```python
from build123d import *

# Parameters (mm, degrees)
F0_R         = 38.1
F0_R_2       = 22.86
F1_DEPTH     = 127
F4_DEPTH     = 80.011
F5_T4_DEPTH  = 27.2677982704
F5_S5_R      = 38.1
F5_T6_DEPTH  = 15
F5_S7_R      = 22.86
F5_T8_DEPTH  = 15
F5_T12_DEPTH = 27.2677982704
F5_S13_R     = 38.1
F5_T14_DEPTH = 15
F5_S15_R     = 22.86
F5_T16_DEPTH = 15
F5_T17_DEPTH = 27.2653813946
F5_T19_DEPTH = 27.2653813946


# Not quite as in the source:
# - a fillet or chamfer that OpenCascade refuses, or shapes differently, is made with other operations: its cross-section is extruded or revolved along the edge and cut away or added


with BuildPart() as f1:
    # F0 (on Top) → F1 (new body)
    with BuildSketch(Plane.XY):
        Circle(F0_R)
        Circle(F0_R_2, mode=Mode.SUBTRACT)
    extrude(amount=F1_DEPTH)

    # F3 (on offset) → F4 (cut, through all)
    with BuildSketch(Plane.XZ.offset(41.91)):
        with BuildLine():
            Line((1.3741332924, 44.0691516455), (0, 44.0691516455))
            Line((0, 44.0691516455), (0, 27.1781024958))
            Line((0, 27.1781024958), (0, -6.6039958037))
            Line((0, -6.6039958037), (38.1, -6.6039958037))
            Line((38.1, -6.6039958037), (38.1, 27.1781024958))
            Line((38.1, 27.1781024958), (18.242812226, 27.1781024958))
            ThreePointArc((18.242812226, 27.1781024958), (15.5282171859, 27.7875908663), (13.3347289514, 29.4990556395))
            Line((13.3347289514, 29.4990556395), (1.3741332924, 44.0691516455))
        make_face()
        with BuildLine():
            Line((0, 44.0691516455), (-1.3741332924, 44.0691516455))
            Line((-1.3741332924, 44.0691516455), (-13.3347289514, 29.4990556395))
            ThreePointArc((-13.3347289514, 29.4990556395), (-15.5282171859, 27.7875908663), (-18.242812226, 27.1781024958))
            Line((-18.242812226, 27.1781024958), (-38.1, 27.1781024958))
            Line((-38.1, 27.1781024958), (-38.1, -6.6039958037))
            Line((-38.1, -6.6039958037), (0, -6.6039958037))
            Line((0, -6.6039958037), (0, 27.1781024958))
            Line((0, 27.1781024958), (0, 44.0691516455))
        make_face()
        with BuildLine():
            Line((38.1, 60.9602007953), (38.1, 77.9781024958))
            Line((38.1, 77.9781024958), (1.27, 77.9781024958))
            Line((1.27, 77.9781024958), (1.2895432809, 77.9542953638))
            Line((1.2895432809, 77.9542953638), (13.3347289514, 63.281153939))
            ThreePointArc((13.3347289514, 63.281153939), (15.5282171859, 61.5696891658), (18.242812226, 60.9602007953))
            Line((18.242812226, 60.9602007953), (38.1, 60.9602007953))
        make_face()
        with BuildLine():
            Line((-38.1, 77.9781024958), (-38.1, 60.9602007953))
            Line((-38.1, 60.9602007953), (-18.242812226, 60.9602007953))
            ThreePointArc((-18.242812226, 60.9602007953), (-15.5282171859, 61.5696891658), (-13.3347289514, 63.281153939))
            Line((-13.3347289514, 63.281153939), (-1.2895432809, 77.9542953638))
            Line((-1.2895432809, 77.9542953638), (-1.27, 77.9781024958))
            Line((-1.27, 77.9781024958), (-38.1, 77.9781024958))
        make_face()
        Polygon((-38.1, 131.2988996506), (-38.1, 77.9781024958), (-1.27, 77.9781024958), (-1.2391987117, 77.9781024958), (-0.1262114529, 77.9781024958), (0, 77.9781024958), (1.2391987117, 77.9781024958), (1.27, 77.9781024958), (38.1, 77.9781024958), (38.1, 80.6030047561), (38.1, 131.2988996506), align=None)
    extrude(amount=-F4_DEPTH, mode=Mode.SUBTRACT)

    # F5: fillet of radius 5.08 on 6 edges, made by hand


with BuildPart() as f5_tool2:
    # F5_s3 → F5_t4 (new body)
    with BuildSketch(Plane.XZ.offset(44.0808363055)):
        with BuildLine():
            ThreePointArc((-1.0281164884, 44.0691516455), (1.1435595437, 43.5815609491), (2.8983501313, 42.2123891305))
            Line((2.8983501313, 42.2123891305), (1.3741332924, 44.0691516455))
            Line((1.3741332924, 44.0691516455), (-1.0281164884, 44.0691516455))
        make_face()
    extrude(amount=-F5_T4_DEPTH)

    # F5_s5 → F5_t6 (intersect, symmetric)
    with BuildSketch(Plane.XY.offset(43.1)):
        Circle(F5_S5_R)
    extrude(amount=F5_T6_DEPTH, both=True, mode=Mode.INTERSECT)

    # F5_s7 → F5_t8 (cut, symmetric)
    with BuildSketch(Plane.XY.offset(43.1)):
        Circle(F5_S7_R)
    extrude(amount=F5_T8_DEPTH, both=True, mode=Mode.SUBTRACT)


with BuildPart() as f1_1:
    add(f1.part)

    # F5_t1: union F5_tool2
    add(f5_tool2.part)


with BuildPart() as f5_tool10:
    # F5_s11 → F5_t12 (new body)
    with BuildSketch(Plane.XZ.offset(44.0808363055)):
        with BuildLine():
            ThreePointArc((-2.8983501313, 42.2123891305), (-1.1435595437, 43.5815609491), (1.0281164884, 44.0691516455))
            Line((1.0281164884, 44.0691516455), (-1.3741332924, 44.0691516455))
            Line((-1.3741332924, 44.0691516455), (-2.8983501313, 42.2123891305))
        make_face()
    extrude(amount=-F5_T12_DEPTH)

    # F5_s13 → F5_t14 (intersect, symmetric)
    with BuildSketch(Plane.XY.offset(43.1)):
        Circle(F5_S13_R)
    extrude(amount=F5_T14_DEPTH, both=True, mode=Mode.INTERSECT)

    # F5_s15 → F5_t16 (cut, symmetric)
    with BuildSketch(Plane.XY.offset(43.1)):
        Circle(F5_S15_R)
    extrude(amount=F5_T16_DEPTH, both=True, mode=Mode.SUBTRACT)


with BuildPart() as f1_2:
    add(f1_1.part)

    # F5_t9: union F5_tool10
    add(f5_tool10.part)

    # F5_s18 → F5_t17 (cut)
    with BuildSketch(Plane.XZ.offset(16.8190705077)):
        with BuildLine():
            ThreePointArc((2.7942168389, 76.1213399807), (1.0394262513, 77.4905117994), (-1.1322497808, 77.9781024958))
            Line((-1.1322497808, 77.9781024958), (1.27, 77.9781024958))
            Line((1.27, 77.9781024958), (2.7942168389, 76.1213399807))
        make_face()
        with BuildLine():
            ThreePointArc((1.1322497808, 77.9781024958), (-1.0394262513, 77.4905117994), (-2.7942168389, 76.1213399807))
            Line((-2.7942168389, 76.1213399807), (-1.27, 77.9781024958))
            Line((-1.27, 77.9781024958), (1.1322497808, 77.9781024958))
        make_face()
    extrude(amount=F5_T17_DEPTH, mode=Mode.SUBTRACT)

    # F5_s20 → F5_t19 (cut)
    with BuildSketch(Plane.XZ.offset(-44.0844519023)):
        with BuildLine():
            ThreePointArc((-1.1322497808, 77.9781024958), (1.0394262513, 77.4905117994), (2.7942168389, 76.1213399807))
            Line((2.7942168389, 76.1213399807), (1.27, 77.9781024958))
            Line((1.27, 77.9781024958), (-1.1322497808, 77.9781024958))
        make_face()
        with BuildLine():
            ThreePointArc((-2.7942168389, 76.1213399807), (-1.0394262513, 77.4905117994), (1.1322497808, 77.9781024958))
            Line((1.1322497808, 77.9781024958), (-1.27, 77.9781024958))
            Line((-1.27, 77.9781024958), (-2.7942168389, 76.1213399807))
        make_face()
    extrude(amount=F5_T19_DEPTH, mode=Mode.SUBTRACT)


solid = f1_2.part
```
For this review, take the finished solid that the model builds, in its own axes (mm). A direction names the side the tool comes from. Give positions to 0.01 mm unless a question says otherwise; leave off trailing zeros. Order: outer loops, then holes, each group sorted by start corner. A loop starts at its lowest first (then second) coordinate and runs counter-clockwise, first axis right, second up.
1) The part is to be moulded in two halves that separate along X. For faces 4 (the face through (-1.62, -30.496, 43.324)), 5 (the face through (-28, 0, 27.178)), 6 (the face through (-15.564, 24.58, 61.553)), 7 (the face through (1.561, -30.286, 77.206)), say which applies: released by +X, released by -X, zero draft, split by the parting line, or undercut.
2) For faces 1 (the face through (28, 0, 60.96)), 2 (the face through (1.58, -30.5, 43.35)), 3 (the face through (-8.14, -28.42, 69.61)), list the 3-axis set-ups (+Z, -Z, +X, -X, +Y, -Y) from which the entire face can be reached by the end or side of a thin tool; tool diameter is ignored.
3) Take a section at C-C (z = 48). Give the boundary of the cut face in (x, y).
4) Take a section at A-A (y = 0). Give the boundary of the cut face in (x, z).
5) Take a section at D-D (x = -31). Give the boundary of the cut face in (y, z), then the cut area to 3 significant figures.
6) Insertion check: pin 1 (4 mm diameter, centred on x = 9, z = 46.5, fed in from +Y); pin 2 (8 mm diameter, centred on y = -2, z = 49, fed in from +X); pin 3 (1.5 mm diameter, centred on y = 25, z = 39.5, fed in from +X); pin 4 (6 mm diameter, centred on x = -28, y = 14.5, fed in from +Z). Each pin has a flat end and moves straight along its axis. Give the tip position at first contact, or say it passes through.
7) Take a section at B-B (x = -5). Give the boundary of the cut face in (y, z), then the cut area to 3 significant figures.
8) Wall thickness on line 1 (X direction, y = 0, z = 38); line 2 (X direction, y = -24.5, z = 39): over which ranges is each line inside the solid? List them lowest first.
Derived:
1. face 4: undercut
1. face 5: zero draft
1. face 6: released by -X
1. face 7: released by +X
2. face 1: +Z, +X, +Y, -Y
2. face 2: -Z, +Y, -Y
2. face 3: +Z, -X, +Y, -Y
3. outline: circle Ø76.2 at (0, 0); hole circle Ø45.72 at (0, 0)
4. outline: (-38.1, 27.18) - (-22.86, 27.18) - (-22.86, 60.96) - (-38.1, 60.96) - close; (22.86, 27.18) - (38.1, 27.18) - (38.1, 60.96) - (22.86, 60.96) - close
5. outline: (-22.15, 27.18) - (22.15, 27.18) - (22.15, 60.96) - (-22.15, 60.96) - close
5. area: 1,500 mm2
6. pin 1: stops at y = 37.45
6. pin 2: stops at x = 38.1
6. pin 3: stops at x = 29.39
6. pin 4: stops at z = 60.96
7. outline: (-37.77, 39.65) - (-22.31, 39.65) - (-22.31, 73.43) - (-37.77, 73.43) - close; (22.31, 39.65) - (37.77, 39.65) - (37.77, 73.43) - (22.31, 73.43) - close
7. area: 1,040 mm2
8. line 1: x = -38.1 to -22.86, 22.86 to 38.1
8. line 2: x = -29.18 to -5.54, 5.54 to 29.18
